For this review, take the finished solid that the model builds, in its own axes (mm). Round coordinates to 2 decimals unless told otherwise and drop trailing zeros. Order: outer loops, then holes, each group sorted by start corner. A loop starts at its lowest first (then second) coordinate and runs counter-clockwise, first axis right, second up.
from build123d import *

# Parameters (mm, degrees)
BOSS_EXTRUDE1_DEPTH = 5.7
SKETCH2_R           = 3.95
CUT_EXTRUDE1_DEPTH  = 10


with BuildPart() as part:
    # Sketch1 → Boss-Extrude1 (new body)
    with BuildSketch(Plane(origin=(0, 0, 0), x_dir=(0, 0, -1), z_dir=(1, 0, 0))):
        Polygon((-140.35, 82.95), (-140.35, 107.95), (140.35, 107.95), (140.35, 82.95), (146.05, 82.95), (146.05, 32.15), (140.35, 32.15), (140.35, -32.15), (146.05, -32.15), (146.05, -82.95), (140.35, -82.95), (140.35, -107.95), (-140.35, -107.95), (-140.35, -82.95), (-146.05, -82.95), (-146.05, -32.15), (-140.35, -32.15), (-140.35, 32.15), (-146.05, 32.15), (-146.05, 82.95), align=None)
    extrude(amount=BOSS_EXTRUDE1_DEPTH)

    # Sketch2 → Cut-Extrude1 (cut)
    with BuildSketch(Plane(origin=(5.7, 0, 0), x_dir=(0, 0, -1), z_dir=(1, 0, 0))):
        with Locations((105.2625, -79.970674176)):
            Circle(SKETCH2_R)
    extrude(amount=-CUT_EXTRUDE1_DEPTH, mode=Mode.SUBTRACT)


solid = part.part
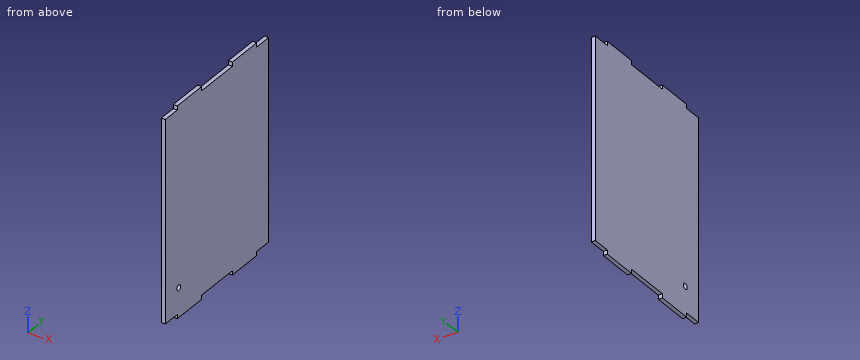
(1) Add section A-A on x = 2.15. Give the boundary of the cut face in (y, z), plus the area to 3 significant figures.
(2) Add section B-B on y = 29. Give the boundary of the cut face in (x, z), plus the area to 3 significant figures.
(3) Clearance check with flat-ended pins moving along their axes: P1, Ø3, axis at x = 2, z = -143.5, coming from the +Y side; P2, Ø3, axis at x = 3, z = 144.5, coming from the -Y side; P3, Ø3, axis at x = 4, y = -96, coming from the -Z side; P4, Ø7, axis at y = -79.97, z = -105.26, coming from the -X side. State where each tip first meets the part, or that it passes through.
(4) Wall thickness on L1, parallel to Z at x = 1.95, y = -26: over which ranges is the line inside the solid? List them lowest first.
Here are the results:
1. outline: (-107.95, -140.35) - (-82.95, -140.35) - (-82.95, -146.05) - (-32.15, -146.05) - (-32.15, -140.35) - (32.15, -140.35) - (32.15, -146.05) - (82.95, -146.05) - (82.95, -140.35) - (107.95, -140.35) - (107.95, 140.35) - (82.95, 140.35) - (82.95, 146.05) - (32.15, 146.05) - (32.15, 140.35) - (-32.15, 140.35) - (-32.15, 146.05) - (-82.95, 146.05) - (-82.95, 140.35) - (-107.95, 140.35) - close; hole circle Ø7.9 at (-79.97, -105.26)
1. area: 61,700 mm2
2. outline: (0, -140.35) - (5.7, -140.35) - (5.7, 140.35) - (0, 140.35) - close
2. area: 1,600 mm2
3. P1: stops at y = 82.95
3. P2: stops at y = -82.95
3. P3: stops at z = -140.35
3. P4: passes through
4. L1: z = -140.35 to 140.35
